For this review, take the finished solid that the model builds, in its own axes (mm). Face numbers are marked on the shaded views. A direction names the side the tool comes from. Round coordinates to 2 decimals unless told otherwise and drop trailing zeros. Write each loop counter-clockwise with the first axis right and the second up, starting at its lowest first coordinate (ties: lowest second). Pieces come first, ordered by that corner, then holes. Notation, with made-up numbers: (62, 45.25) -> (85, 45.25) arc R29 cw to (85, 82.25) -> close; hole circle Ø6 at (79, -17.5). An arc over 180 degrees is marked (long way). Answer in a Markdown table with one row per item.
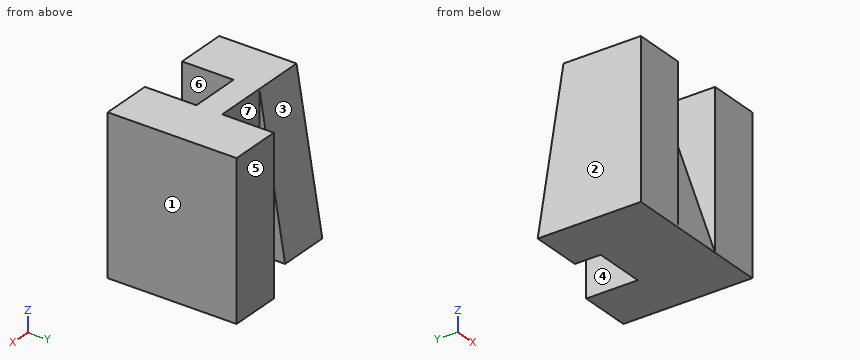
from build123d import *

# Parameters (mm, degrees)
SKETCH1_W           = 6
SKETCH1_H           = 6
BOSS_EXTRUDE1_DEPTH = 5
SKETCH2_W           = 6
SKETCH2_H           = 2
CUT_EXTRUDE1_DEPTH  = 1
CUT_EXTRUDE2_DEPTH  = 2


with BuildPart() as part:
    # Sketch1 → Boss-Extrude1 (new body)
    with BuildSketch(Plane(origin=(0, 0, 0), x_dir=(1, 0, 0), z_dir=(0, 1, 0))):
        Rectangle(SKETCH1_W, SKETCH1_H)
    extrude(amount=BOSS_EXTRUDE1_DEPTH)

    # Sketch2 → Cut-Extrude1 (cut, symmetric)
    with BuildSketch(Plane(origin=(0, 0, 0), x_dir=(0, 0, -1), z_dir=(1, 0, 0))):
        Polygon((3, 0), (-3, 2), (-3, 0), align=None)
        with Locations((0, 4)):
            Rectangle(SKETCH2_W, SKETCH2_H)
    extrude(amount=CUT_EXTRUDE1_DEPTH, both=True, mode=Mode.SUBTRACT)

    # Sketch3 → Cut-Extrude2 (cut)
    with BuildSketch(Plane.ZY.offset(3)):
        Polygon((-3, 4), (3, 3), (3, 5), (-3, 5), align=None)
    extrude(amount=-CUT_EXTRUDE2_DEPTH, mode=Mode.SUBTRACT)


solid = part.part
1) Consider section A-A on y = 3.35. State the section outline as (x, z) points, then the cut area to 3 significant figures.
Solved:
| item | result |
|---|---|
| outline | (-3, -3) -> (-1, -3) -> (-1, 0.9) -> (-3, 0.9) -> close; (1, -3) -> (3, -3) -> (3, 3) -> (1, 3) -> close |
| area | 19.8 mm² |
2) Consider section B-B on z = -2.5. State the section outline as (x, y) points.
Solved:
| item | result |
|---|---|
| outline | (-3, 0) -> (-1, 0) -> (-1, 0.17) -> (1, 0.17) -> (1, 0) -> (3, 0) -> (3, 5) -> (1, 5) -> (1, 3) -> (-1, 3) -> (-1, 3.92) -> (-3, 3.92) -> close |
3) Consider section D-D on x = -2.1. State the section outline as (y, z) points.
Solved:
| item | result |
|---|---|
| outline | (0, -3) -> (4, -3) -> (3, 3) -> (0, 3) -> close |
4) For the marked faces 5, 6 and 7, list the 3-axis set-ups (+Z, -Z, +X, -X, +Y, -Y) from which the entire face can be reached by the end or side of a thin tool; tool diameter is ignored.
Solved:
| item | result |
|---|---|
| face 5 | +Z, -Z, +X, -X, +Y |
| face 6 | +Z, -Y |
| face 7 | +Z, -Z, +Y |
5) Consider section C-C on y = 0.5. State the section outline as (x, z) points.
Solved:
| item | result |
|---|---|
| outline | (-3, -3) -> (3, -3) -> (3, 3) -> (1, 3) -> (1, -1.5) -> (-1, -1.5) -> (-1, 3) -> (-3, 3) -> close |
6) Clearance check with flat-ended pins moving along their axes: pin 1 Ø1 at (x, z) = (0, 0) entering from -Y; pin 2 Ø1.5 at (x, z) = (-2.5, -1) entering from +Y. State where each tip first meets the part, or that it passes through.
Solved:
| item | result |
|---|---|
| pin 1 | y = 0.83 |
| pin 2 | y = 3.79 |
7) Mouldability with a two-part tool opening along X and no side actions: class the marked faces 1, 2, 3 and 4 as pulls with the +X half, pulls with the -X half, needs draft (parallel to the pull), parting line crosses it, or undercut.
Solved:
| item | result |
|---|---|
| face 1 | pulls with the +X half |
| face 2 | pulls with the -X half |
| face 3 | needs draft |
| face 4 | undercut |
8) For line 1 (X direction, y = 0.3, z = 1); line 2 (X direction, y = 4.4, z = -1); line 3 (Y direction, x = -1.3, z = -2.25) (3 decimals), list the stretches that pass through material, from the lowest coordinate up. Write a range as [from, to].
Solved:
| item | result |
|---|---|
| line 1 | [-3, -1], [1, 3] |
| line 2 | [1, 3] |
| line 3 | [0, 3.875] |
